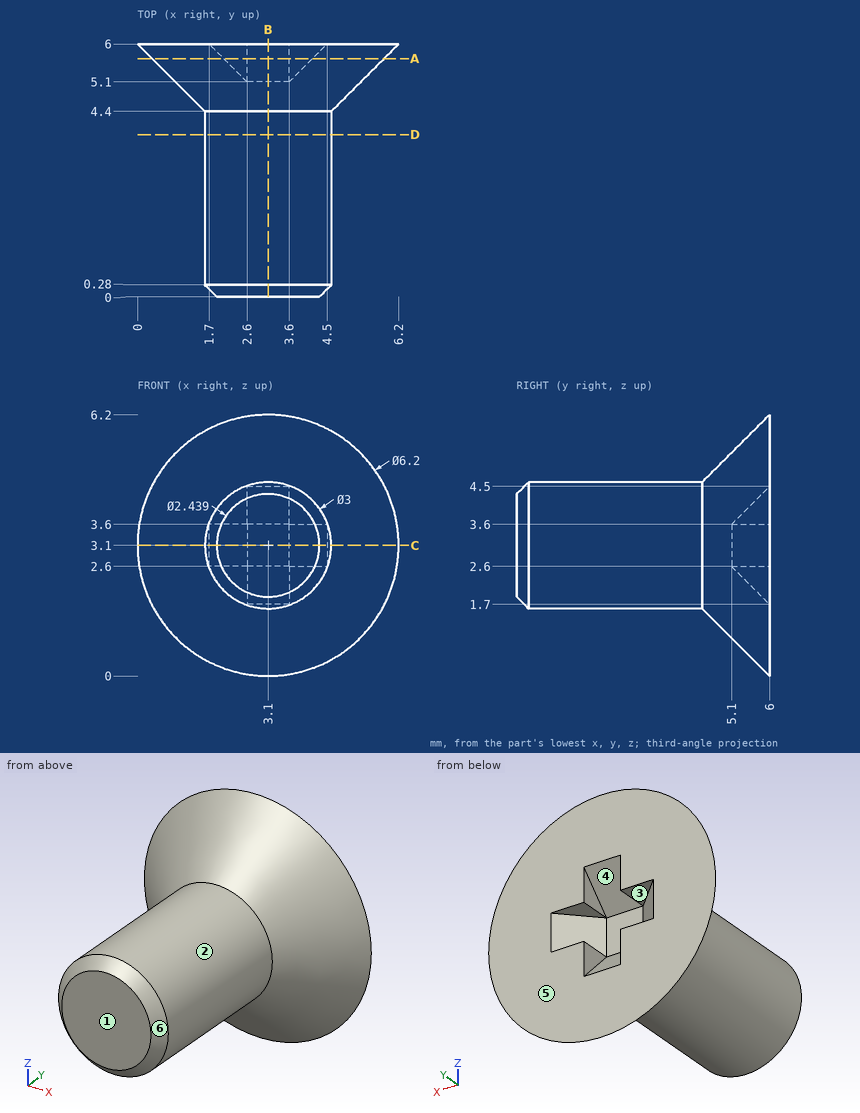
Study the drawing (mm; zero at the part's minimum x, y, z) and answer. A direction names the side the tool comes from. Give positions to 0.01 mm unless a question says otherwise; leave off trailing zeros. Order: outer loops, then holes, each group sorted by start corner. A loop starts at its lowest first (then second) coordinate and runs counter-clockwise, first axis right, second up.
1. Section D-D, the plane y = 3.85 is taken. Determine the outline of the cut face in (x, z).
Result sheet:
outline: circle Ø3 at (3.1, 3.1)
2. Each of these flat-tipped pins is pushed along its axis until it touches: P1, Ø1, axis at x = 5, z = 4, coming from the -Y side; P2, Ø0.7, axis at x = 2.5, y = 5.5, coming from the +Z side (1 decimal); P3, Ø1.5, axis at x = 3.5, z = 0.5, coming from the -Y side. Where does it stop, or does it pass through?
Result sheet:
P1: stops at y = 4.5
P2: stops at z = 6
P3: stops at y = 4.78
3. For the marked faces 1, 2 and 3, determine the directions among +Z, -Z, +X, -X, +Y, -Y from which every point of the face is accessible in a straight line to the end or side of a thin tool.
Result sheet:
face 1: +Z, -Z, +X, -X, -Y
face 2: -Y
face 3: +Y
4. Section B-B, the plane x = 3.1 is taken. Determine the outline of the cut face in (y, z).
Result sheet:
outline: (0, 1.88) - (0.28, 1.6) - (4.4, 1.6) - (6, 0) - (6, 1.7) - (5.1, 2.6) - (5.1, 3.6) - (6, 4.5) - (6, 6.2) - (4.4, 4.6) - (0.28, 4.6) - (0, 4.32) - close
5. Straight lines are drawn through the part: L1, parallel to Y at x = 2.75, z = 3.25; L2, parallel to Z at x = 3, y = 5.6; L3, parallel to X at y = 5.75, z = 4 (1 decimal). For each, find the intervals that lie inside material, in ascending order.
Result sheet:
L1: y = 0 to 5.1
L2: z = 0.4 to 2.1, 4.1 to 5.8
L3: x = 0.4 to 2.6, 3.6 to 5.8
6. Section A-A, the plane y = 5.65 is taken. Determine the outline of the cut face in (x, z).
Result sheet:
outline: circle Ø5.5 at (3.1, 3.1); hole (2.05, 2.6) - (2.6, 2.6) - (2.6, 2.05) - (3.6, 2.05) - (3.6, 2.6) - (4.15, 2.6) - (4.15, 3.6) - (3.6, 3.6) - (3.6, 4.15) - (2.6, 4.15) - (2.6, 3.6) - (2.05, 3.6) - close
7. Section C-C, the plane z = 3.1 is taken. Determine the outline of the cut face in (x, y).
Result sheet:
outline: (0, 6) - (1.6, 4.4) - (1.6, 0.28) - (1.88, 0) - (4.32, 0) - (4.6, 0.28) - (4.6, 4.4) - (6.2, 6) - (4.5, 6) - (3.6, 5.1) - (2.6, 5.1) - (1.7, 6) - close
8. The mould has two halves that part along Z. Classify the marked faces 4, 5 and 6: released by +Z, released by -Z, zero draft, split by the parting line, or undercut.
Result sheet:
face 4: undercut
face 5: zero draft
face 6: split by the parting line
